from build123d import *

# Parameters (mm, degrees)
RESSALTO_EXTRUS_O1_DEPTH = 2.7
ESBO_O1_6_R              = 4.825
RESSALTO_EXTRUS_O2_DEPTH = 4.3
ESBO_O4_R                = 3
CORTE_EXTRUS_O1_DEPTH    = 3.65
ESBO_O5_R                = 2
CORTE_EXTRUS_O2_DEPTH    = 3.65


with BuildPart() as part:
    # Esbo_o1 → Ressalto-extrus_o1 (new body)
    with BuildSketch(Plane(origin=(0, 0, 0), x_dir=(1, 0, 0), z_dir=(0, 1, 0))):
        with BuildLine():
            Line((0.495762712, 6.481066219), (29.824152542, 4.23762022))
            ThreePointArc((29.824152542, 4.23762022), (33.746903927, -0.162194428), (29.5, -4.25))
            Line((29.5, -4.25), (0.498520942, -6.48085464))
            ThreePointArc((0.498520942, -6.48085464), (-6.499999853, -0.001383166), (0.495762712, 6.481066219))
        make_face()
    extrude(amount=RESSALTO_EXTRUS_O1_DEPTH)

    # Esbo_o1_6 → Ressalto-extrus_o2 (add)
    with BuildSketch(Plane(origin=(0, 0, 0), x_dir=(1, 0, 0), z_dir=(0, 1, 0))):
        with Locations(Location((0, 0, 0), (0, 0, 270))):
            Circle(ESBO_O1_6_R)
    extrude(amount=-RESSALTO_EXTRUS_O2_DEPTH)

    # Esbo_o4 → Corte-extrus_o1 (cut)
    with BuildSketch(Plane(origin=(0, 2.7, 0), x_dir=(1, 0, 0), z_dir=(0, 1, 0))):
        with Locations(Location((0, 0, 0), (0, 0, 270))):
            Circle(ESBO_O4_R)
    extrude(amount=-CORTE_EXTRUS_O1_DEPTH, mode=Mode.SUBTRACT)

    # Esbo_o5 → Corte-extrus_o2 (cut)
    with BuildSketch(Plane(origin=(0, -0.95, 0), x_dir=(1, 0, 0), z_dir=(0, 1, 0))):
        with Locations(Location((0, 0, 0), (0, 0, 270))):
            Circle(ESBO_O5_R)
    extrude(amount=-CORTE_EXTRUS_O2_DEPTH, mode=Mode.SUBTRACT)


solid = part.part
Source: CAD feature listing. Evaluate the final solid. Frame: model axes, mm. A direction names the side the tool comes from. Round coordinates to 2 decimals unless told otherwise and drop trailing zeros. Order: outer loops, then holes, each group sorted by start corner. A loop starts at its lowest first (then second) coordinate and runs counter-clockwise, first axis right, second up. Notation, with made-up numbers: (-37, 43) - (6, 43) arc R21 ccw to (6, 63) - close; hole circle Ø7 at (-6, 57.25). An arc over 180 degrees is marked (long way). Use a Markdown table: item, result. Add a question column.
1. Set-up query: faces 4 (the cylindrical face through (4.784, -2.12, -0.628)), 5 (the flat face through (14.955, 1.331, -5.375)), 6 (the flat face through (-1, -0.95, 2)). Return all of +Z, -Z, +X, -X, +Y, -Y with unobstructed straight access to the full face (end or side cutting, diameter ignored); none if empty.
2. Mould query, pull axis X, two halves, no side actions, for faces 1 (the flat face through (14, 2.7, 0)), 2 (the flat face through (15.2, 1.33, 5.35)), 3 (the cylindrical face through (-2, -3, 0)). Classes: +X half, -X half, draft (parallel to the pull), parting line (faces both ways), or undercut.
3. Section query B-B (y = 1.25). Return the cut outline in (x, z).
4. Line query: probe 1 along X at (y, z) = (-3.15, 0) (3 decimals); probe 2 along X at (y, z) = (2, 0); probe 3 along Y at (x, z) = (11, 2.5). Output: solid intervals per line, ascending.
5. Section query D-D (y = -2). Return the cut outline in (x, z) (3 decimals), then the cut area to 3 significant figures.
6. Section query A-A (x = 0). Return the cut outline in (y, z) (3 decimals), then the cut area to 3 significant figures.
7. Section query C-C (z = 0.5). Return the cut outline in (x, y), then the cut area to 3 significant figures.
Derived:
| question | item | result |
|---|---|---|
| 1 | face 4 | -Y |
| 1 | face 5 | -Z, +X, +Y, -Y |
| 1 | face 6 | +Y |
| 2 | face 1 | draft |
| 2 | face 2 | +X half |
| 2 | face 3 | undercut |
| 3 | outline | (0.5, -6.48) - (29.82, -4.24) arc R4.25 ccw to (29.5, 4.25) - (0.5, 6.48) arc R6.5 ccw (long way) to start; hole circle Ø6 at (0, 0) |
| 4 | probe 1 | -4.825 to -2, 2 to 4.825 |
| 4 | probe 2 | -6.5 to -3, 3 to 33.75 |
| 4 | probe 3 | 0 to 2.7 |
| 5 | outline | circle Ø9.65 at (0, 0); hole circle Ø4 at (0, 0) |
| 5 | area | 60.6 mm2 |
| 6 | outline | (-4.3, -4.825) - (0, -4.825) - (0, -6.5) - (2.7, -6.5) - (2.7, -3) - (-0.95, -3) - (-0.95, -2) - (-4.3, -2) - close; (-4.3, 2) - (-0.95, 2) - (-0.95, 3) - (2.7, 3) - (2.7, 6.5) - (0, 6.5) - (0, 4.825) - (-4.3, 4.825) - close |
| 6 | area | 41.3 mm2 |
| 7 | outline | (-6.48, 0) - (-4.8, 0) - (-4.8, -4.3) - (-1.94, -4.3) - (-1.94, -0.95) - (-2.96, -0.95) - (-2.96, 2.7) - (-6.48, 2.7) - close; (1.94, -4.3) - (4.8, -4.3) - (4.8, 0) - (33.72, 0) - (33.72, 2.7) - (2.96, 2.7) - (2.96, -0.95) - (1.94, -0.95) - close |
| 7 | area | 115 mm2 |
